For this review, take the finished solid that the model builds, in its own axes (mm). A direction names the side the tool comes from. Coordinates: 2 decimals unless noted, no trailing zeros. Loops run counter-clockwise (first coordinate to the right, second up) from the corner with the lowest first, then second, coordinate; pieces in that order, holes last. Notation, with made-up numbers: (48.5, 36.5) - (104.5, 36.5) arc R12 cw to (104.5, 59.5) - close; hole circle Ø6 at (89, 38). An arc over 180 degrees is marked (long way). Use one line per item in the form item = value. Start each with the question number.
1. To check wall thickness, follow probe 1 along Z at (x, y) = (10, 2.3); probe 2 along X at (y, z) = (2.3, -18); probe 3 along Y at (x, z) = (3.5, -18). State the ranges of each line that lie inside material, in increasing order.
2. Add section B-B on z = -5. Give the boundary of the cut face in (x, y).
3. Add section D-D on x = 2.5. Give the boundary of the cut face in (y, z).
4. For pin 1 Ø0.8 at (y, z) = (2, -7.5) entering from +X; pin 2 Ø0.8 at (x, y) = (2, 2) entering from +Z; pin 3 Ø0.8 at (x, y) = (5, 2) entering from -Z, all flat-tipped, find the tip position at first contact; note any pin that passes through.
5. Machinability: for faces 4 (the face through (14.5, 1, 0)), 5 (the face through (-14.5, 1, 0)), 6 (the face through (0, 2, 20.5)), 7 (the face through (0, 1, -21.5)), 8 (the face through (0, 1, 21.5)), which of the approach directions +Z, -Z, +X, -X, +Y, -Y give a long, thin tool a straight path to every point of the face, cutting with its end or side? Answer none if there is none.
6. Add section A-A on x = -13. Give the boundary of the cut face in (y, z), and give its area (4 significant figures).
7. Draft analysis for pull direction X (two halves, no side actions). For faces 1 (the face through (0, 2, -20.5)), 2 (the face through (-22.5, -1, 0)), 3 (the face through (0, -1, -22.5)), state which applies: +X half, -X half, draft (parallel to the pull), parting line (faces both ways), or undercut.
8. Add section C-C on y = 0.55. Give the boundary of the cut face in (x, z).
Autodesk Inventor part; units mm, degrees
ref_plane "YZ Plane" through (0, 0, 0) normal (1, 0, 0) x (0, 1, 0)
ref_plane "XZ Plane" through (0, 0, 0) normal (0, 1, 0) x (-1, 0, 0)
ref_plane "XY Plane" through (0, 0, 0) normal (0, 0, 1) x (1, 0, 0)
sketch "Sketch1" plane through (0, 0, 0) normal (0, 1, 0) x (-1, 0, 0)
  line L0 (-22.5, 22.5) -> (22.5, 22.5)
  line L1 (22.5, 22.5) -> (22.5, -22.5)
  line L2 (22.5, -22.5) -> (-22.5, -22.5)
  line L3 (-22.5, -22.5) -> (-22.5, 22.5)
  line L4 (-22.5, 22.5) -> (22.5, -22.5) construction
  line L5 (22.5, 22.5) -> (-22.5, -22.5) construction
  line L6 (-14.5, 21.5) -> (14.5, 21.5)
  line L7 (14.5, 21.5) -> (14.5, -21.5)
  line L8 (14.5, -21.5) -> (-14.5, -21.5)
  line L9 (-14.5, -21.5) -> (-14.5, 21.5)
  line L10 (-14.5, 21.5) -> (14.5, -21.5) construction
  line L11 (14.5, 21.5) -> (-14.5, -21.5) construction
  point P0 (0, 0)
  dimension "d0" = 45
  dimension "d1" = 45
  dimension "d2" = 29
  dimension "d3" = 43
extrude "Extrusion1" add sketch "Sketch1" against normal blind 1.6 contours L0 L1 L2 L3 | L6 L7 L8 L9
extrude "Extrusion2" add sketch "Sketch1" along normal blind 2.5 contours L6 L7 L8 L9
sketch "Sketch2" plane through (0, 2.5, 0) normal (0, 1, 0) x (1, 0, 0)
  line L0 (12, -20.5) -> (-12, -20.5)
  line L1 (-12, -20.5) -> (-12, 20.5)
  line L2 (-12, 20.5) -> (12, 20.5)
  line L3 (12, 20.5) -> (12, -20.5)
  line L4 (12, -20.5) -> (-12, 20.5) construction
  line L5 (-12, -20.5) -> (12, 20.5) construction
  point P0 (0, 0)
  dimension "d8" = 24
  dimension "d9" = 41
extrude "Extrusion3" cut sketch "Sketch2" against normal blind 1
properties part number "LCD5110"
Conclusion:
q1.probe_1 = -21.5 to -20.5, 20.5 to 21.5
q1.probe_2 = -14.5 to -12, 12 to 14.5
q1.probe_3 = -1.6 to 1.5
q2.outline = (-22.5, -1.6) - (22.5, -1.6) - (22.5, 0) - (14.5, 0) - (14.5, 2.5) - (12, 2.5) - (12, 1.5) - (-12, 1.5) - (-12, 2.5) - (-14.5, 2.5) - (-14.5, 0) - (-22.5, 0) - close
q3.outline = (-1.6, -22.5) - (0, -22.5) - (0, -21.5) - (2.5, -21.5) - (2.5, -20.5) - (1.5, -20.5) - (1.5, 20.5) - (2.5, 20.5) - (2.5, 21.5) - (0, 21.5) - (0, 22.5) - (-1.6, 22.5) - close
q4.pin_1 = 14.5
q4.pin_2 = 21.5
q4.pin_3 = -21.5
q5.face_4 = +Z, -Z, +X, +Y
q5.face_5 = +Z, -Z, -X, +Y
q5.face_6 = +Y
q5.face_7 = -Z, +X, -X, +Y
q5.face_8 = +Z, +X, -X, +Y
q6.outline = (-1.6, -22.5) - (0, -22.5) - (0, -21.5) - (2.5, -21.5) - (2.5, 21.5) - (0, 21.5) - (0, 22.5) - (-1.6, 22.5) - close
q6.area = 179.5 mm^2
q7.face_1 = undercut
q7.face_2 = -X half
q7.face_3 = draft
q8.outline = (-14.5, -21.5) - (14.5, -21.5) - (14.5, 21.5) - (-14.5, 21.5) - close
